Part model, mm, in its own coordinate system. A direction names the side the tool comes from. Give positions to 0.01 mm unless a question says otherwise; leave off trailing zeros. Write each loop counter-clockwise with the first axis right and the second up, starting at its lowest first coordinate (ties: lowest second). Pieces come first, ordered by that corner, then holes.
```python
from build123d import *

# Parameters (mm, degrees)
F0_R            = 50.2948420816
F1_DEPTH        = 25
F2_R            = 21.9350719346
F3_DEPTH        = 25
F5_DEPTH        = 25
F5_COPIES_COUNT = 15


# Not quite as in the source:
# - a pattern or mirror of a feature is missing from the dataset's text; its kind, count and spacing are read off the source's solid


with BuildPart() as f1:
    # F0 (on Front) → F1 (new body)
    with BuildSketch(Plane.XZ):
        Circle(F0_R)
    extrude(amount=F1_DEPTH)

    # F2 (on face) → F3 (cut)
    with BuildSketch(Plane.XZ.offset(25)):
        Circle(F2_R)
    extrude(amount=-F3_DEPTH, mode=Mode.SUBTRACT)

    # F4 (on Front) → F5 (join)
    with BuildSketch(Plane.XZ):
        with BuildLine():
            Line((0, 63), (-8.656896714, 49.5442153969))
            ThreePointArc((-8.656896714, 49.5442153969), (0, 50.2948420816), (8.656896714, 49.5442153969))
            Line((8.656896714, 49.5442153969), (0, 63))
        make_face()
    f5 = extrude(amount=F5_DEPTH)

    # F5_copies: F5 ×15 about axis
    f5_copies_axis = Axis((0, 0, 0), (0, 1, 0))
    for i in range(1, F5_COPIES_COUNT):
        add(f5.rotate(f5_copies_axis, i * 360 / F5_COPIES_COUNT))


solid = f1.part
```
1) Wall check: L1, parallel to Z at x = 0, y = -10.25; L2, parallel to X at y = -2.75, z = 50; L3, parallel to Z at x = 52.5, y = -12.25 (3 decimals). Give the ranges that are in metal, low to high.
Answers follow:
L1: z = -50.29 to -21.94, 21.94 to 63
L2: x = -26.79 to -14.1, -8.36 to 8.36, 14.1 to 26.79
L3: z = -31.599 to -27.5, -11.705 to 1.566, 10.389 to 21.421
2) 3-axis set-ups, long thin cutter, end or side, ignore diameter. For faces 1 (the face through (50.022, -12.325, 5.232)), 2 (the face through (39.033, -12.325, 40.888)), 3 (the face through (-44.744, -12.325, 34.545)): which of +Z, -Z, +X, -X, +Y, -Y reach the whole face in a straight line?
Answers follow:
face 1: +X, +Y, -Y
face 2: +Z, +Y, -Y
face 3: -X, +Y, -Y
3) Two-plate mould, pull along Z, no slides. Class faces 4 (the face through (-10.43, -12.32, 49.2)), 5 (the face through (-50.017, -12.325, 5.283)), 6 (the face through (44.685, -12.325, 34.329)), 7 (the face through (29.47, -12.32, -48.03)): +Z half, -Z half, draft (parallel to the pull), parting line (faces both ways), or undercut.
Answers follow:
face 4: +Z half
face 5: undercut
face 6: undercut
face 7: -Z half
4) Saw through at A-A, the plane x = -52. Write the cut outline in (y, z).
Answers follow:
outline: (-25, -31.62) - (0, -31.62) - (0, -26.53) - (-25, -26.53) - close; (-25, -11.96) - (0, -11.96) - (0, 1.97) - (-25, 1.97) - close; (-25, 9.78) - (0, 9.78) - (0, 21.55) - (-25, 21.55) - close
5) Saw through at B-B, the plane z = 0. Write the cut outline in (x, y), then the cut area to 3 significant figures.
Answers follow:
outline: (-54.45, -25) - (-21.94, -25) - (-21.94, 0) - (-54.45, 0) - close; (21.94, -25) - (54.45, -25) - (54.45, 0) - (21.94, 0) - close
area: 1,630 mm2
6) Pin check, flat tips, straight feed: pin 1 Ø10 at (y, z) = (-19, 2.5) entering from -X; pin 2 Ø1 at (y, z) = (-4, 2) entering from -X; pin 3 Ø3 at (x, y) = (13, -12.5) entering from -Z; pin 4 Ø12 at (x, z) = (32.5, 37.5) entering from +Y. Stop position of each tip, or through.
Answers follow:
pin 1: stops at x = -57.57
pin 2: stops at x = -52.58
pin 3: stops at z = -61.62
pin 4: stops at y = 0
7) Saw through at D-D, the plane z = -19. Write the cut outline in (x, y), then the cut area to 3 significant figures.
Answers follow:
outline: (-48.12, -25) - (-10.96, -25) - (-10.96, 0) - (-48.12, 0) - close; (10.96, -25) - (48.12, -25) - (48.12, 0) - (10.96, 0) - close
area: 1,860 mm2
8) Saw through at C-C, the plane z = 54. Write the cut outline in (x, y).
Answers follow:
outline: (-26.17, -25) - (-20.2, -25) - (-20.2, 0) - (-26.17, 0) - close; (-5.79, -25) - (5.79, -25) - (5.79, 0) - (-5.79, 0) - close; (20.2, -25) - (26.17, -25) - (26.17, 0) - (20.2, 0) - close
